CAD build for the part. Positions are in the model's coordinates, mm. A direction names the side the tool comes from. Give positions to 0.01 mm unless a question says otherwise; leave off trailing zeros. Loops run counter-clockwise (first coordinate to the right, second up) from the corner with the lowest first, then second, coordinate; pieces in that order, holes last. Notation, with made-up numbers: M 6.25,69 L 65.25,69 A16 cw 65.25,96 Z; hole C 15.5,-28 d6. An arc over 180 degrees is marked long. Answer as CSV lines item,"result".
```python
from build123d import *

# Parameters (mm, degrees)
BASE_FLANGE1_DEPTH = 38.1
SKETCH6_R          = 2.4892
CUT_EXTRUDE1_DEPTH = 245.358693113


# Sheet-metal steps are written as plain solids
with BuildPart() as part:
    # Sketch1 → Base-Flange1 (new, symmetric)
    with BuildSketch(Plane.XY):
        with BuildLine():
            Line((-120.015, 0), (-120.015, 23.0505))
            ThreePointArc((-120.015, 23.0505), (-119.326847382, 24.711847382), (-117.6655, 25.4))
            Line((-117.6655, 25.4), (117.6655, 25.4))
            ThreePointArc((117.6655, 25.4), (119.326847382, 24.711847382), (120.015, 23.0505))
            Line((120.015, 23.0505), (120.015, 0))
            Line((120.015, 0), (118.4275, 0))
            Line((118.4275, 0), (118.4275, 23.0505))
            ThreePointArc((118.4275, 23.0505), (118.204315367, 23.589315367), (117.6655, 23.8125))
            Line((117.6655, 23.8125), (-117.6655, 23.8125))
            ThreePointArc((-117.6655, 23.8125), (-118.204315367, 23.589315367), (-118.4275, 23.0505))
            Line((-118.4275, 23.0505), (-118.4275, 0))
            Line((-118.4275, 0), (-120.015, 0))
        make_face()
    extrude(amount=BASE_FLANGE1_DEPTH, both=True)

    # Sketch6 → Cut-Extrude1 (cut, through all)
    with BuildSketch(Plane.ZY.offset(120.015)):
        with Locations((-31.75, 11.52525)):
            Circle(SKETCH6_R)
        with Locations((31.75, 11.52525)):
            Circle(SKETCH6_R)
    extrude(amount=-CUT_EXTRUDE1_DEPTH, mode=Mode.SUBTRACT)


solid = part.part
```
Q1. Cut at A-A (y = 6.25). Write the cut outline in (x, z) (1 decimal).
Solution:
outline,"M -120,-38.1 L -118.4,-38.1 L -118.4,38.1 L -120,38.1 Z; M 118.4,-38.1 L 120,-38.1 L 120,38.1 L 118.4,38.1 Z"
Q2. Cut at C-C (z = -6). Write the cut outline in (x, y) (1 decimal).
Solution:
outline,"M -120,0 L -118.4,0 L -118.4,23.1 A0.8 cw -117.7,23.8 L 117.7,23.8 A0.8 cw 118.4,23.1 L 118.4,0 L 120,0 L 120,23.1 A2.3 ccw 117.7,25.4 L -117.7,25.4 A2.3 ccw -120,23.1 Z"
Q3. Mould opens along Y. For faces 3 (the flat face through (-2, 25.4, 1)), 4 (the cylindrical face through (119.21, 11.635, 29.263)), 5 (the flat face through (2, 23.812, 1)), 6 (the flat face through (1, 25, -38.1)) say: released by +Y, released by -Y, zero draft, split by the parting line, or undercut.
Solution:
face 3,"released by +Y"
face 4,"undercut"
face 5,"released by -Y"
face 6,"zero draft"
Q4. Which spindle directions (+Z, -Z, +X, -X, +Y, -Y) get a long thin tool onto all of the face, cutting with end or side? Do faces 1 (the cylindrical face through (119.21, 11.635, -34.237)), 2 (the flat face through (118.428, 11, 1)). Say none if no direction does.
Solution:
face 1,"+X, -X"
face 2,"+Z, -Z, -Y"
Q5. Cut at D-D (x = -90). Write the cut outline in (y, z), and give its area (3 significant figures).
Solution:
outline,"M 23.81,-38.1 L 25.4,-38.1 L 25.4,38.1 L 23.81,38.1 Z"
area,"121 mm²"
Q6. Wall check: line 1 (X direction, y = 9.75, z = -28.5) (1 decimal); line 2 (Y direction, x = -119, z = 31); line 3 (Y direction, x = 119.2, z = 31.75). Give the ranges that are in metal, low to high. Write a range as [from, to].
Solution:
line 1,"x = [-120, -118.4], [118.4, 120]"
line 2,"y = [0, 9.15], [13.9, 24.98]"
line 3,"y = [0, 9.04], [14.01, 24.83]"
Q7. Pin check, flat tip, straight feed: P1, Ø6, axis at x = -79, y = 23, coming from the +Z side. Stop position of the tip, or through.
Solution:
P1,"stops at z = 38.1"
Q8. Cut at B-B (z = 31.75). Write the cut outline in (x, y) (1 decimal), and give its area (3 significant figures).
Solution:
outline,"M -120,0 L -118.4,0 L -118.4,9 L -120,9 Z; M -120,14 L -118.4,14 L -118.4,23.1 A0.8 cw -117.7,23.8 L 117.7,23.8 A0.8 cw 118.4,23.1 L 118.4,14 L 120,14 L 120,23.1 A2.3 ccw 117.7,25.4 L -117.7,25.4 A2.3 ccw -120,23.1 Z; M 118.4,0 L 120,0 L 120,9 L 118.4,9 Z"
area,"439 mm²"
